Verification items for this drawing (mm, ordinates from the low corner). A direction names the side the tool comes from. Coordinates: 2 decimals unless noted, no trailing zeros. Loops run counter-clockwise (first coordinate to the right, second up) from the corner with the lowest first, then second, coordinate; pieces in that order, holes last. Notation, with made-up numbers: M 10,51 L 45,51 A14 ccw 45,78 Z; hole C -4,-39.5 d11. An arc over 180 degrees is marked long. One line per question, with ' | ' between items. Start each with the question number.
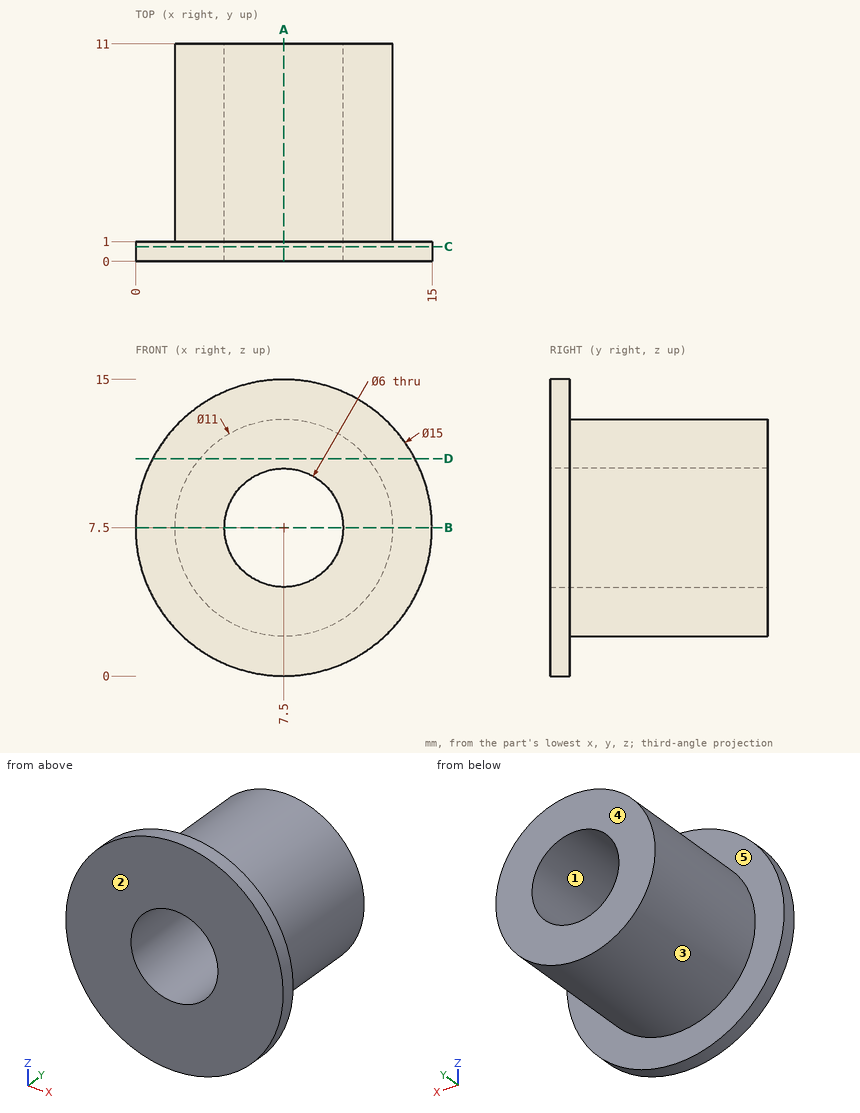
1. Sectioned sample at D-D (z = 11). Record the cut outline in (x, y), and give its area (3 significant figures).
2. Tool access check on the marked faces 4 and 5. Record the directions out of +Z, -Z, +X, -X, +Y, -Y that give a thin tool (end or side, any length) a straight path to the whole face; none if there is none.
3. Depth check by flat-ended pin: pin 1 Ø1.5 at (x, y) = (11, 1) entering from +Z; pin 2 Ø1 at (y, z) = (2, 8.5) entering from +X. Enter the tip coordinate at first touch or a pass-through.
4. Thickness scan on line 1 (X direction, y = 5, z = 7.5); line 2 (X direction, y = 9.5, z = 5.75); line 3 (Z direction, x = 10.25, y = 2.75). Record the ranges inside material, lowest first.
5. Sectioned sample at C-C (y = 0.75). Record the cut outline in (x, z), and give its area (3 significant figures).
6. Draft check along X on the marked faces 1, 2 and 3. Enter one of: +X half, -X half, draft (parallel to the pull), parting line (faces both ways), or undercut.
7. Sectioned sample at A-A (x = 7.5). Record the cut outline in (y, z), and give its area (3 significant figures).
8. Sectioned sample at B-B (z = 7.5). Record the cut outline in (x, y).
Result:
1) outline: M 0.87,0 L 14.13,0 L 14.13,1 L 11.74,1 L 11.74,11 L 3.26,11 L 3.26,1 L 0.87,1 Z | area: 98.1 mm2
2) face 4: +Z, -Z, +X, -X, +Y | face 5: +Y
3) pin 1: stops at z = 14.48 | pin 2: stops at x = 12.98
4) line 1: x = 2 to 4.5, 10.5 to 13 | line 2: x = 2.29 to 5.06, 9.94 to 12.71 | line 3: z = 2.74 to 6.3, 8.7 to 12.26
5) outline: C 7.5,7.5 d15; hole C 7.5,7.5 d6 | area: 148 mm2
6) face 1: undercut | face 2: draft | face 3: parting line
7) outline: M 0,0 L 1,0 L 1,2 L 11,2 L 11,4.5 L 0,4.5 Z; M 0,10.5 L 11,10.5 L 11,13 L 1,13 L 1,15 L 0,15 Z | area: 59.0 mm2
8) outline: M 0,0 L 4.5,0 L 4.5,11 L 2,11 L 2,1 L 0,1 Z; M 10.5,0 L 15,0 L 15,1 L 13,1 L 13,11 L 10.5,11 Z
